```python
from build123d import *

# Parameters (mm, degrees)
F1_DEPTH = 6.35
F3_T     = 6.35


# Not quite as in the source:
# - a feature names something its author has since deleted; it is built from what else it names


with BuildPart() as f1:
    # F0 (on Top) → F1 (new body)
    with BuildSketch(Plane.XY):
        Polygon((-47.7481111884, 27.6977252215), (-74.0418732166, -56.7705929279), (16.344493255, -59.0262524784), align=None)
    extrude(amount=F1_DEPTH)

    # F3
    f3_openings = [f1.faces().sort_by_distance(p)[0] for p in [
        (-35.148497, -29.366373, 6.35),
    ]]
    offset(amount=F3_T, openings=f3_openings, kind=Kind.INTERSECTION)


solid = f1.part
```
Geometry check sheet. Reference: the model listing, model coordinates, mm. A direction names the side the tool comes from. Coordinates: 2 decimals unless noted, no trailing zeros. Loops run counter-clockwise (first coordinate to the right, second up) from the corner with the lowest first, then second, coordinate; pieces in that order, holes last. Notation, with made-up numbers: (-38.75, 17.5) - (11.25, 17.5) arc R18 ccw to (11.25, 39.5) - close; hole circle Ø1 at (75, 5). An arc over 180 degrees is marked (long way). One line per item, written item: value. Start each with the question number.
(1) Tool access check on faces 1 (the flat face through (-66.118, -9.95, -0.089)), 2 (the flat face through (-60.711, -13.945, 3.131)). Record the directions out of +Z, -Z, +X, -X, +Y, -Y that give a thin tool (end or side, any length) a straight path to the whole face; none if there is none.
(2) Cross-section at A-A on z = 3.25. Enter the section's corners in (x, y).
(3) Cross-section at D-D on z = -3. Enter the section's corners in (x, y), plus the area to 3 significant figures.
(4) Cross-section at B-B on x = 1. Enter the section's corners in (y, z).
(5) Cross-section at C-C on y = -9.5. Enter the section's corners in (x, z).
(6) Mould release check, pull along Y, two halves, no side actions. Record for faces 3 (the flat face through (-15.253, -16.271, 3.131)), 4 (the flat face through (-9.9, -12.83, -0.09)), 5 (the flat face through (-40, -35, -6.35)), 6 (the flat face through (-40, -34, 0)): released by +Y, released by -Y, zero draft, split by the parting line, or undercut.
(7) Depth check by flat-ended pin: P1, Ø1, axis at x = -25.5, z = -2.5, coming from the -Y side; P2, Ø3, axis at x = -26.5, z = -2, coming from the +Y side; P3, Ø5, axis at x = -2, z = 3, coming from the -Y side. Enter the tip coordinate at first touch or a pass-through.
(8) Material ranges on line 1 (Z direction, x = -40.5, y = -1.5); line 2 (Y direction, x = 3.5, z = 1); line 3 (X direction, y = -13.5, z = 3.5), recorded low to high. Write a range as [from, to].
Results below:
1. face 1: +Z, -Z, -X, +Y
1. face 2: +Z
2. outline: (-82.6, -62.91) - (29.17, -65.7) - (-50.09, 41.55) - close; hole (-74.04, -56.77) - (16.34, -59.03) - (-47.75, 27.7) - close
3. outline: (-82.6, -62.91) - (29.17, -65.7) - (-50.09, 41.55) - close
3. area: 5,880 mm2
4. outline: (-65, -6.35) - (-27.58, -6.35) - (-27.58, 6.35) - (-38.26, 6.35) - (-38.26, 0) - (-58.64, 0) - (-58.64, 6.35) - (-65, 6.35) - close
5. outline: (-65.98, -6.35) - (-12.36, -6.35) - (-12.36, 6.35) - (-20.26, 6.35) - (-20.26, 0) - (-59.33, 0) - (-59.33, 6.35) - (-65.98, 6.35) - close
6. face 3: undercut
6. face 4: released by +Y
6. face 5: zero draft
6. face 6: undercut
7. P1: stops at y = -64.35
7. P2: stops at y = 11.66
7. P3: stops at y = -64.98
8. line 1: z = [-6.35, 0]
8. line 2: y = [-65.06, -58.71], [-41.65, -30.96]
8. line 3: x = [-67.22, -60.57], [-17.3, -9.41]
